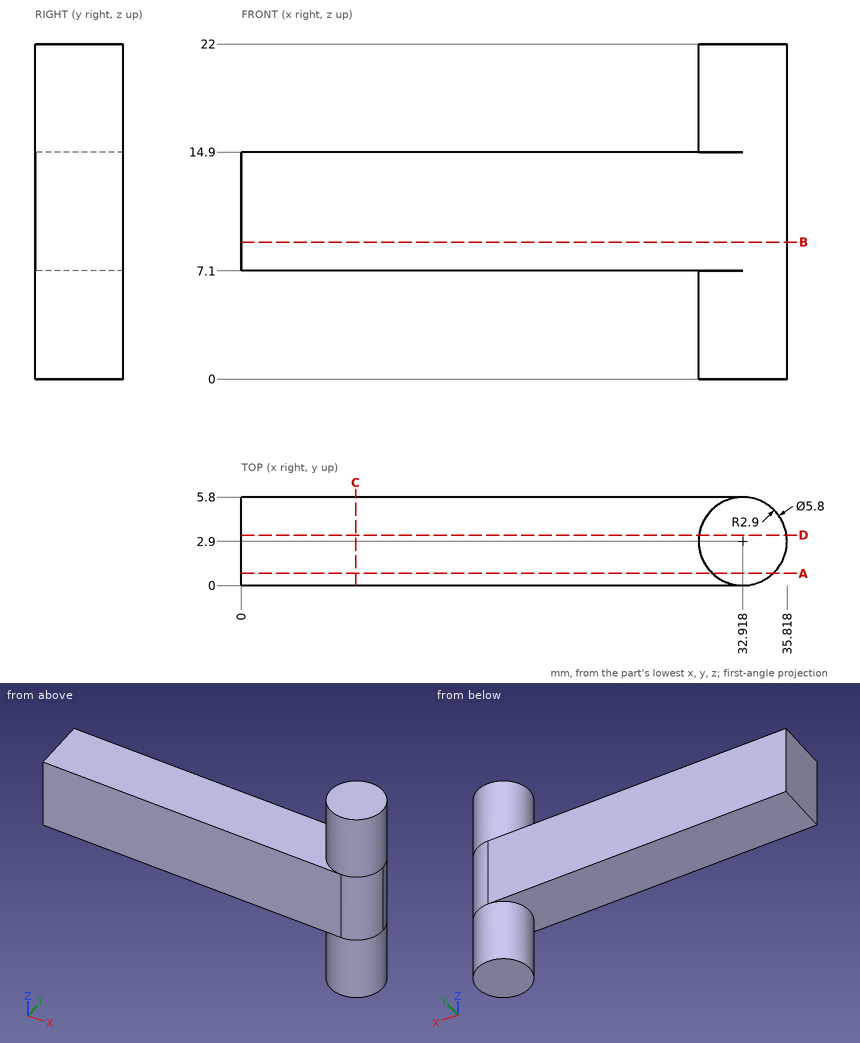
Design review of the part shown in the three views and the two pictorial views. Dimensions are in mm from the part's minimum x, y and z. Give positions to 0.01 mm unless a question says otherwise; leave off trailing zeros. Loops run counter-clockwise (first coordinate to the right, second up) from the corner with the lowest first, then second, coordinate; pieces in that order, holes last. Notation, with made-up numbers: (-9.5, 62.5) -> (14.5, 62.5) arc R22 cw to (14.5, 95.5) -> close; hole circle Ø4 at (-26, 65.5). An arc over 180 degrees is marked (long way). Put each result on its own line as item: value. Start each with the question number.
1. Wall thickness on probe 1 along Z at (x, y) = (14, 0.7); probe 2 along X at (y, z) = (2.4, 14.5) (1 decimal); probe 3 along X at (y, z) = (1.6, 7.5): over which ranges is each line inside the solid? List them lowest first.
2. We need section D-D on y = 3.3. State the section outline as (x, z) points (1 decimal), then the cut area to 3 significant figures.
3. We need section C-C on x = 7.5. State the section outline as (y, z) points.
4. We need section A-A on y = 0.8. State the section outline as (x, z) points, then the cut area to 3 significant figures.
5. We need section B-B on z = 9. State the section outline as (x, y) points, then the cut area to 3 significant figures.
6. Clearance check with flat-ended pins moving along their axes: P1, Ø3, axis at x = 23.5, y = 2.5, coming from the -Z side; P2, Ø1, axis at x = 13.5, y = 3.5, coming from the +Z side. State where each tip first meets the part, or that it passes through.
Determined:
1. probe 1: 7.1 to 14.9
1. probe 2: 0 to 35.8
1. probe 3: 0 to 35.51
2. outline: (0, 7.1) -> (30, 7.1) -> (30, 0) -> (35.8, 0) -> (35.8, 22) -> (30, 22) -> (30, 14.9) -> (0, 14.9) -> close
2. area: 361 mm^2
3. outline: (0, 7.1) -> (5.8, 7.1) -> (5.8, 14.9) -> (0, 14.9) -> close
4. outline: (0, 7.1) -> (30.92, 7.1) -> (30.92, 0) -> (34.92, 0) -> (34.92, 22) -> (30.92, 22) -> (30.92, 14.9) -> (0, 14.9) -> close
4. area: 329 mm^2
5. outline: (0, 0) -> (32.92, 0) arc R2.9 ccw to (32.92, 5.8) -> (0, 5.8) -> close
5. area: 204 mm^2
6. P1: z = 7.1
6. P2: z = 14.9
